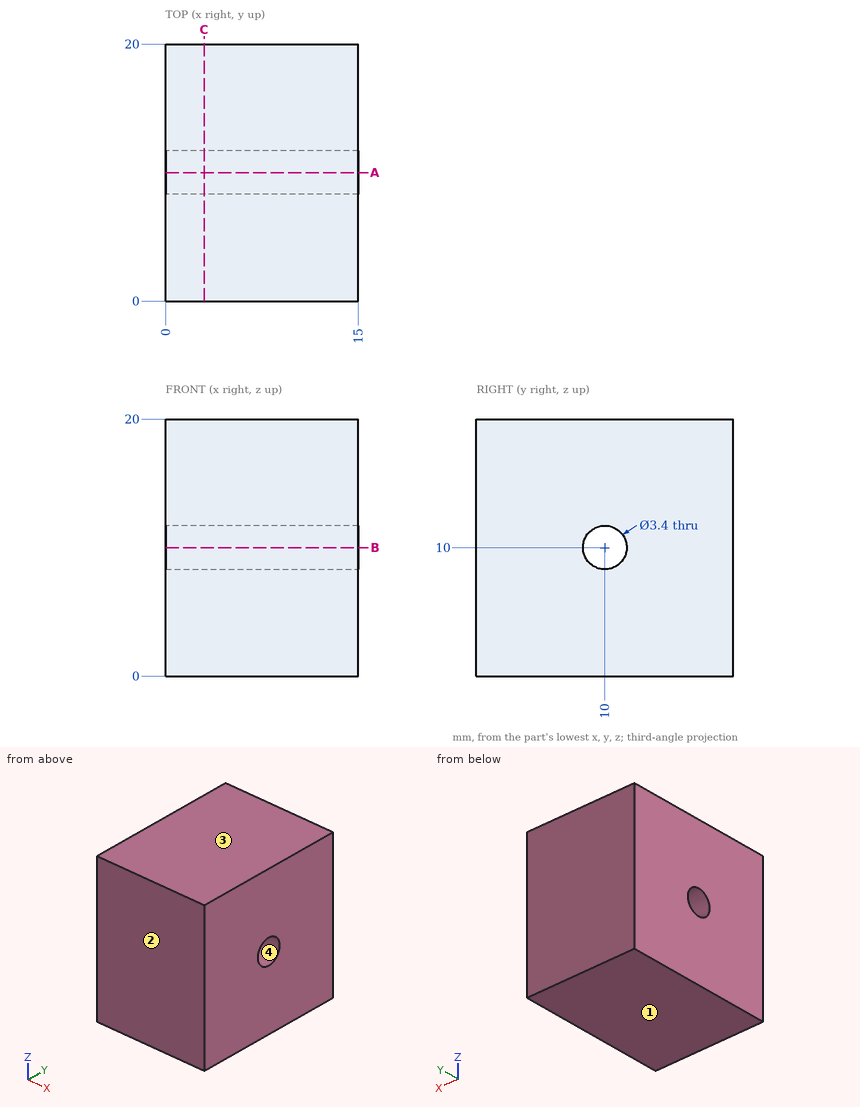
Input: dimensioned drawing with shaded views. Units: mm. Origin: part minimum x, y, z. Give positions to 0.01 mm unless a question says otherwise; leave off trailing zeros. Loops run counter-clockwise (first coordinate to the right, second up) from the corner with the lowest first, then second, coordinate; pieces in that order, holes last. Notation, with made-up numbers: M 75,19 L 82,19 A19 cw 82,55 Z; hole C -15.75,38.25 d5. An arc over 180 degrees is marked long. Put each result on its own line as item: value. Start each with the question number.
1) Pull-direction query (Z, two-part tool) for the marked faces 1, 2, 3 and 4; classes: pulls with the +Z half, pulls with the -Z half, needs draft (parallel to the pull), parting line crosses it, or undercut.
2) Cut plane C-C (x = 3). Output: boundary loops of the cut face in (y, z).
3) Cut plane A-A (y = 10). Output: boundary loops of the cut face in (x, z), then the cut area to 3 significant figures.
4) Contact query for a flat-ended pin moving along its axis: pin 1 (4 mm diameter, centred on y = 10, z = 10, fed in from +X). Output: stop coordinate, or through.
5) Ray query, line 1 along Y through (x, z) = (11.75, 10); line 2 along Z through (x, y) = (10.25, 8.5). Return the intervals inside material, ascending.
Verdict:
1. face 1: pulls with the -Z half
1. face 2: needs draft
1. face 3: pulls with the +Z half
1. face 4: undercut
2. outline: M 0,0 L 20,0 L 20,20 L 0,20 Z; hole C 10,10 d3.4
3. outline: M 0,0 L 15,0 L 15,8.3 L 0,8.3 Z; M 0,11.7 L 15,11.7 L 15,20 L 0,20 Z
3. area: 249 mm2
4. pin 1: x = 15
5. line 1: 0 to 8.3, 11.7 to 20
5. line 2: 0 to 9.2, 10.8 to 20
